The model under review builds one solid part; all positions refer to its coordinate system, in mm. Face numbers are marked on the shaded views. A direction names the side the tool comes from. Coordinates: 2 decimals unless noted, no trailing zeros. Order: outer loops, then holes, each group sorted by start corner. A loop starts at its lowest first (then second) coordinate and runs counter-clockwise, first axis right, second up. Notation, with made-up numbers: M -33,-19.5 L 13,-19.5 A35 ccw 13,12.5 Z; hole C 33,-17.75 d7. An arc over 180 degrees is marked long. Answer in a Markdown table with one row per item.
from build123d import *

# Parameters (mm, degrees)
F2_DEPTH       = 304.8
F3_W           = 1079.5
F3_H           = 1079.5
F4_DEPTH       = 50.8
F5_SIZE        = 25.4
F7_R           = 63.5
F8_DEPTH       = 50.8
F9_W           = 779.78
F9_H           = 558.8
F9_W_2         = 754.38
F9_H_2         = 533.4
F9_R           = 63.5
F10_DEPTH      = 50.8
F12_DEPTH      = 254
F12_DEPTH_BACK = 635


with BuildPart() as f2:
    # F1 (on face) → F2 (new body)
    with BuildSketch(Plane.XY):
        Polygon((539.75, -825.5), (539.75, 254), (488.95, 254), (488.95, -698.5), (-488.95, -698.5), (-488.95, 254), (-539.75, 254), (-539.75, -825.5), align=None)
    extrude(amount=F2_DEPTH)

    # F3 (on Top) → F4 (join)
    with BuildSketch(Plane.XY):
        with Locations((0, -285.75)):
            Rectangle(F3_W, F3_H)
    extrude(amount=F4_DEPTH)

    # F5
    f5_edges = [f2.edges().sort_by_distance(p)[0] for p in [
        (0, -825.5, 0),
        (-539.75, -825.5, 152.4),
        (0, -825.5, 304.8),
        (539.75, -825.5, 152.4),
    ]]
    chamfer(f5_edges, length=F5_SIZE)

    # F7 (on face) → F8 (cut, through all)
    with BuildSketch(Plane.XY.offset(50.8)):
        Circle(F7_R)
    extrude(amount=-F8_DEPTH, mode=Mode.SUBTRACT)

    # F9 (on face) → F10 (cut, through all)
    with BuildSketch(Plane.XY.offset(50.8)):
        with Locations((-97.79, -63.5)):
            Rectangle(F9_W, F9_H)
        with Locations((-97.79, -63.5)):
            Rectangle(F9_W_2, F9_H_2, mode=Mode.SUBTRACT)
        with Locations((-97.79, -63.5)):
            Rectangle(F9_W_2, F9_H_2)
        Circle(F9_R, mode=Mode.SUBTRACT)
    extrude(amount=-F10_DEPTH, mode=Mode.SUBTRACT)

    # F11 (on Front) → F12 (cut, two sides)
    with BuildSketch(Plane.XZ) as f12_sk:
        Polygon((557.425588846, 76.2), (557.425588846, 152.4), (557.425588846, 228.6), (532.025588846, 228.6), (532.025588846, 215.9), (538.375588846, 215.9), (538.375588846, 222.25), (551.075588846, 222.25), (551.075588846, 152.4), (551.075588846, 82.55), (538.375588846, 82.55), (538.375588846, 88.9), (532.025588846, 88.9), (532.025588846, 76.2), align=None)
        Polygon((-532.025588846, 88.9), (-538.375588846, 88.9), (-538.375588846, 82.55), (-551.075588846, 82.55), (-551.075588846, 152.4), (-551.075588846, 222.25), (-538.375588846, 222.25), (-538.375588846, 215.9), (-532.025588846, 215.9), (-532.025588846, 228.6), (-557.425588846, 228.6), (-557.425588846, 152.4), (-557.425588846, 76.2), (-532.025588846, 76.2), align=None)
    extrude(amount=-F12_DEPTH, mode=Mode.SUBTRACT)
    extrude(f12_sk.sketch, amount=F12_DEPTH_BACK, mode=Mode.SUBTRACT)


solid = f2.part
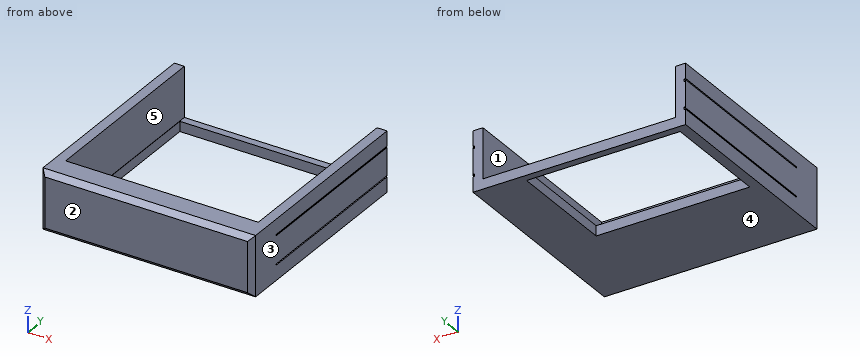
(1) Take a section at A-A (x = -383.5). Write out the cut boundary in (y, z).
Report:
| item | result |
|---|---|
| outline | M -825.5,25.4 L -800.1,0 L -342.9,0 L -342.9,50.8 L -698.5,50.8 L -698.5,304.8 L -800.1,304.8 L -825.5,279.4 Z; M 215.9,0 L 254,0 L 254,50.8 L 215.9,50.8 Z |
(2) Take a section at D-D (x = 342). Write out the cut boundary in (y, z), then the cut area to 3 significant figures.
Report:
| item | result |
|---|---|
| outline | M -825.5,25.4 L -800.1,0 L 254,0 L 254,50.8 L -698.5,50.8 L -698.5,304.8 L -800.1,304.8 L -825.5,279.4 Z |
| area | 86,500 mm^2 |
(3) To check wall thickness, follow line 1 (X direction, y = -177, z = 186.5); line 2 (Y direction, x = -480, z = 34); line 3 (X direction, y = -0.5, z = 39.5). State the ranges of each line that lie inside material, in increasing order. Write a range as [from, to].
Report:
| item | result |
|---|---|
| line 1 | [-539.75, -488.95], [488.95, 539.75] |
| line 2 | [-825.5, -342.9], [215.9, 254] |
| line 3 | [-539.75, -487.68], [292.1, 539.75] |
(4) Take a section at B-B (y = -665). Write out the cut boundary in (x, z).
Report:
| item | result |
|---|---|
| outline | M -539.75,0 L 539.75,0 L 539.75,304.8 L 488.95,304.8 L 488.95,50.8 L -488.95,50.8 L -488.95,304.8 L -539.75,304.8 Z |
(5) Take a section at C-C (z = 198). Write out the cut boundary in (x, y).
Report:
| item | result |
|---|---|
| outline | M -539.75,-800.1 L -514.35,-825.5 L 514.35,-825.5 L 539.75,-800.1 L 539.75,254 L 488.95,254 L 488.95,-698.5 L -488.95,-698.5 L -488.95,254 L -539.75,254 Z |
(6) Insertion check: P1, Ø8, axis at x = 362, z = 171.5, coming from the +Y side; P2, Ø10, axis at x = 401.5, y = -390.5, coming from the +Z side; P3, Ø4, axis at x = 535, z = 223.5, coming from the +Y side. Each pin has a flat end and moves straight along its axis. Give the tip position at first contact, or say it passes through.
Report:
| item | result |
|---|---|
| P1 | y = -698.5 |
| P2 | z = 50.8 |
| P3 | y = -635 |
(7) Machinability: for the marked faces 4 and 5, which of the approach directions +Z, -Z, +X, -X, +Y, -Y give a long, thin tool a straight path to every point of the face, cutting with its end or side? Answer none if there is none.
Report:
| item | result |
|---|---|
| face 4 | -Z, +X, -X, +Y, -Y |
| face 5 | +Z, +Y |
(8) The part is to be moulded in two halves that separate along X. For the marked faces 1, 2 and 3, say which applies: +X half, -X half, draft (parallel to the pull), parting line (faces both ways), or undercut.
Report:
| item | result |
|---|---|
| face 1 | undercut |
| face 2 | draft |
| face 3 | +X half |
